```python
from build123d import *

# Parameters (mm, degrees)
SKETCH_1_W      = 12
SKETCH_1_H      = 11.3
EXTRUDE_1_DEPTH = 1
SKETCH_2_W      = 1.35
SKETCH_2_H      = 4
EXTRUDE_2_DEPTH = 5.35
SKETCH_3_W      = 1.6
SKETCH_3_H      = 4
EXTRUDE_3_DEPTH = 0.8
SKETCH_4_W      = 1.6
SKETCH_4_H      = 4
EXTRUDE_4_DEPTH = 0.8
FILLET_1_R      = 0.8
FILLET_2_R      = 0.3
SKETCH_5_W      = 1
SKETCH_5_H      = 11.3
EXTRUDE_5_DEPTH = 0.8
SKETCH_6_W      = 1
SKETCH_6_H      = 11.3
EXTRUDE_6_DEPTH = 0.8


with BuildPart() as part:
    # 스케치1 → 보스-돌출1 (new body)
    with BuildSketch(Plane.XY):
        Rectangle(SKETCH_1_W, SKETCH_1_H)
    extrude(amount=EXTRUDE_1_DEPTH)

    # 스케치2 → 보스-돌출2 (add)
    with BuildSketch(Plane.XY.offset(1)):
        with Locations((-5.325, 0)):
            Rectangle(SKETCH_2_W, SKETCH_2_H)
        with Locations((5.325, 0)):
            Rectangle(SKETCH_2_W, SKETCH_2_H)
    extrude(amount=EXTRUDE_2_DEPTH)

    # 스케치3 → 보스-돌출3 (add)
    with BuildSketch(Plane(origin=(-4.65, 0, 0), x_dir=(0, 0, -1), z_dir=(1, 0, 0))):
        with Locations((-5.55, 0)):
            Rectangle(SKETCH_3_W, SKETCH_3_H)
    extrude(amount=EXTRUDE_3_DEPTH)

    # 스케치4 → 보스-돌출4 (add)
    with BuildSketch(Plane.ZY.offset(-4.65)):
        with Locations((5.55, 0)):
            Rectangle(SKETCH_4_W, SKETCH_4_H)
    extrude(amount=EXTRUDE_4_DEPTH)

    # 필렛1
    fillet_1_edges = [part.edges().sort_by_distance(p)[0] for p in [
        (3.85, 0, 6.35),
        (3.85, 0, 4.75),
        (-3.85, 0, 6.35),
        (-3.85, 0, 4.75),
    ]]
    fillet(fillet_1_edges, radius=FILLET_1_R - 0.0001)  # a hair under: the kernel refuses the full size

    # 필렛2
    fillet_2_edges = [part.edges().sort_by_distance(p)[0] for p in [
        (-4.65, 0, 1),
        (4.65, 0, 1),
    ]]
    fillet(fillet_2_edges, radius=FILLET_2_R)

    # 스케치5 → 보스-돌출5 (add)
    with BuildSketch(Plane.ZY.offset(6)):
        with Locations((0.5, 0)):
            Rectangle(SKETCH_5_W, SKETCH_5_H)
    extrude(amount=EXTRUDE_5_DEPTH)

    # 스케치6 → 보스-돌출6 (add)
    with BuildSketch(Plane(origin=(6, 0, 0), x_dir=(0, 0, -1), z_dir=(1, 0, 0))):
        with Locations((-0.5, 0)):
            Rectangle(SKETCH_6_W, SKETCH_6_H)
    extrude(amount=EXTRUDE_6_DEPTH)


solid = part.part
```
Can you work these out from the model? Positions are in its coordinate system, mm. A direction names the side the tool comes from. Coordinates: 2 decimals unless noted, no trailing zeros. Order: outer loops, then holes, each group sorted by start corner. A loop starts at its lowest first (then second) coordinate and runs counter-clockwise, first axis right, second up. Notation, with made-up numbers: (-17, 79) - (31, 79) arc R18 cw to (31, 114) - close; hole circle Ø5 at (80, 12.25). An arc over 180 degrees is marked (long way). Answer in a Markdown table with one row per item.
1. If we mould it in two halves opening along X, with no side actions, what happens to faces 4 (the flat face through (0, 0, 1)), 5 (the flat face through (-6.8, 0.1, 0.5)), 6 (the flat face through (-0.1, 5.65, 0.5)), 7 (the flat face through (6, 0, 4))? For each: pulls with the +X half, pulls with the -X half, needs draft (parallel to the pull), parting line crosses it, or undercut.
Reply:
| item | result |
|---|---|
| face 4 | undercut |
| face 5 | pulls with the -X half |
| face 6 | needs draft |
| face 7 | pulls with the +X half |
2. Suppose I cut it at B-B (x = -5). Please give me the cut outline in (y, z).
Reply:
| item | result |
|---|---|
| outline | (-5.65, 0) - (5.65, 0) - (5.65, 1) - (2, 1) - (2, 6.35) - (-2, 6.35) - (-2, 1) - (-5.65, 1) - close |
3. Suppose I cut it at D-D (z = 5.25). Please give me the cut outline in (x, y), and give its area (3 significant figures).
Reply:
| item | result |
|---|---|
| outline | (-6, -2) - (-3.91, -2) - (-3.91, 2) - (-6, 2) - close; (3.91, -2) - (6, -2) - (6, 2) - (3.91, 2) - close |
| area | 16.7 mm^2 |
4. Suppose I cut it at A-A (z = 4.5). Please give me the cut outline in (x, y), and give its area (3 significant figures).
Reply:
| item | result |
|---|---|
| outline | (-6, -2) - (-4.65, -2) - (-4.65, 2) - (-6, 2) - close; (4.65, -2) - (6, -2) - (6, 2) - (4.65, 2) - close |
| area | 10.8 mm^2 |
5. For pin 1 (1.1 mm diameter, centred on x = 5.5, z = 4, fed in from -Y); pin 2 (3 mm diameter, centred on y = 0.5, z = 5, fed in from +X); pin 3 (5.5 mm diameter, centred on x = 0.5, y = 1, fed in from +Z); pin 4 (2 mm diameter, centred on y = -3.5, z = 3, fed in from +X), each with a flat end and sliding along its axis, tell me the tip position at first contact or that it passes through.
Reply:
| item | result |
|---|---|
| pin 1 | stops at y = -2 |
| pin 2 | stops at x = 6 |
| pin 3 | stops at z = 1 |
| pin 4 | passes through |
6. If I drill on line 1 along X through (y, z) = (-1.5, 4.5); line 2 along Z through (x, y) = (1, 2); line 3 along X through (y, z) = (-0.75, 5.75), over which ranges is the centre line in solid material (lowest first)?
Reply:
| item | result |
|---|---|
| line 1 | x = -6 to -4.65, 4.65 to 6 |
| line 2 | z = 0 to 1 |
| line 3 | x = -6 to -3.88, 3.88 to 6 |
7. For faces 1 (the flat face through (-5, 2, 4)), 2 (the flat face through (-4.65, 0, 3)), 3 (the flat face through (-5, -2, 4)), which set-ups out of +Z, -Z, +X, -X, +Y, -Y let a thin tool reach every point of the face, with its end or its side?
Reply:
| item | result |
|---|---|
| face 1 | +Z, +X, -X, +Y |
| face 2 | +Y, -Y |
| face 3 | +Z, +X, -X, -Y |
